Geometry check sheet. Reference: the model listing, model coordinates, mm. Face numbers are marked on the shaded views. A direction names the side the tool comes from. Give positions to 0.01 mm unless a question says otherwise; leave off trailing zeros. Loops run counter-clockwise (first coordinate to the right, second up) from the corner with the lowest first, then second, coordinate; pieces in that order, holes last.
1. Cross-section at B-B, the plane z = 0. Record the cut outline in (x, y).
2. Go/stop test with flat-tipped pins: pin 1 Ø9 at (y, z) = (13, 7.5) entering from -X; pin 2 Ø8 at (x, y) = (10, 6.5) entering from -Z; pin 3 Ø1.5 at (y, z) = (10, 14.5) entering from +X; pin 4 Ø10 at (x, y) = (30.5, 13.5) entering from +Z. Record where each tip stops, or that it passes through.
3. Cross-section at C-C, the plane y = 15.5. Record the cut outline in (x, z).
4. Cross-section at A-A, the plane x = 0. Record the cut outline in (y, z), plus the area to 3 significant figures.
5. Release check for a two-part mould opening along X. For the marked faces 5, 6, 7 and 8 record: +X half, -X half, draft (parallel to the pull), parting line (faces both ways), or undercut.
6. Material ranges on L1, parallel to X at y = 15.25, z = 4; L2, parallel to Z at x = 2, y = 8.75; L3, parallel to Y at x = -21, z = 10, recorded low to high.
7. Tool access check on the marked faces 1, 2, 3 and 4. Record the directions out of +Z, -Z, +X, -X, +Y, -Y that give a thin tool (end or side, any length) a straight path to the whole face; none if there is none.
8. Cross-section at D-D, the plane x = -24. Record the cut outline in (y, z).
Autodesk Fusion 360 part; units mm, degrees
sketch "Sketch1" plane through (0, 0, 0) normal (0, 1, 0) x (1, 0, 0)
  circle A0 centre (0, 0) radius 40
  line L0 (26.5, -18.7) -> (-26.5, -18.7)
  line L1 (-26.5, -18.7) -> (-26.5, 18.7)
  line L2 (-26.5, 18.7) -> (26.5, 18.7)
  line L3 (26.5, -18.7) -> (-26.5, 18.7) construction
  line L4 (-26.5, -18.7) -> (26.5, 18.7) construction
  line L5 (-28.5, 20.7) -> (28.5, 20.7)
  line L6 (28.5, -20.7) -> (-28.5, -20.7)
  dimension "d1" = 80
  dimension "d2" = 37.4
  dimension "d3" = 53
  dimension "d5" = 37.4
  dimension "d6" = 53
extrude "Extrude1" add sketch "Sketch1" along normal blind 2
sketch "Sketch2" plane through (0, 2, 0) normal (0, 1, 0) x (-1, 0, 0)
  circle A0 centre (0, 0) radius 40
  line L0 (-18.7, 26.5) -> (18.7, 26.5)
  line L1 (18.7, 26.5) -> (18.7, -26.5)
  line L2 (18.7, -26.5) -> (-18.7, -26.5)
  line L3 (-18.7, -26.5) -> (-18.7, 26.5)
  line L4 (-18.7, 26.5) -> (18.7, -26.5) construction
  line L5 (18.7, 26.5) -> (-18.7, -26.5) construction
  line L6 (20.7, 28.5) -> (20.7, -28.5)
  line L7 (20.7, -28.5) -> (-20.7, -28.5)
  line L8 (-20.7, -28.5) -> (-20.7, 28.5)
  line L9 (-20.7, 28.5) -> (20.7, 28.5)
  dimension "d9" = 37.4
  dimension "d10" = 53
  dimension "d11" = -2
extrude "Extrude2" add sketch "Sketch2" along normal blind 16 contours L6 L7 L8 L9
extrude "Extrude3" cut 1 faces at (-6.2333, 2, -8.8333) along direction (0, -1, 0) blind 13
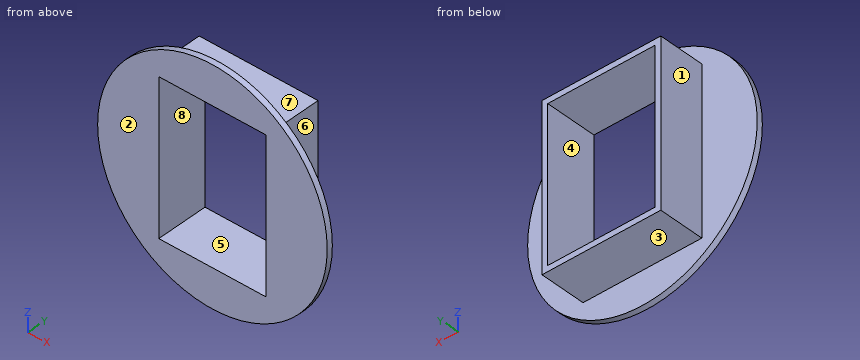
Result:
1. outline: (-40, 0) - (-18.7, 0) - (-18.7, 18) - (-20.7, 18) - (-20.7, 2) - (-40, 2) - close; (18.7, 0) - (40, 0) - (40, 2) - (20.7, 2) - (20.7, 18) - (18.7, 18) - close
2. pin 1: stops at x = -20.7
2. pin 2: stops at z = -28.5
2. pin 3: stops at x = 20.7
2. pin 4: passes through
3. outline: (-20.7, -28.5) - (20.7, -28.5) - (20.7, 28.5) - (-20.7, 28.5) - close; hole (-18.7, -26.5) - (18.7, -26.5) - (18.7, 26.5) - (-18.7, 26.5) - close
4. outline: (0, -40) - (2, -40) - (2, -28.5) - (18, -28.5) - (18, -26.5) - (0, -26.5) - close; (0, 26.5) - (18, 26.5) - (18, 28.5) - (2, 28.5) - (2, 40) - (0, 40) - close
4. area: 118 mm2
5. face 5: undercut
5. face 6: +X half
5. face 7: draft
5. face 8: undercut
6. L1: x = -20.7 to -18.7, 18.7 to 20.7
6. L2: z = -28.5 to -26.5, 26.5 to 28.5
6. L3: y = 0 to 2
7. face 1: +Z, -Z, -X, +Y
7. face 2: +Z, -Z, +X, -X, -Y
7. face 3: -Z, +X, -X, +Y
7. face 4: +Y, -Y
8. outline: (0, -32) - (2, -32) - (2, 32) - (0, 32) - close
